from build123d import *

# Parameters (mm, degrees)
PAD001_DEPTH  = 1
PAD_DEPTH     = 5
SKETCH002_R   = 4.25
SKETCH002_R_2 = 3
SKETCH002_W   = 3
SKETCH002_H   = 16
POCKET_DEPTH  = 5


with BuildPart() as part:
    # Sketch → Pad001 (new body)
    with BuildSketch(Plane.XY):
        with BuildLine():
            Line((0, 67), (0, 0))
            Line((0, 0), (55.315734, 3.5))
            ThreePointArc((55.315734, 3.5), (58.645454, 5.067936), (60, 8.490021))
            Line((60, 8.490021), (60, 58.509979))
            ThreePointArc((60, 58.509979), (58.645454, 61.932064), (55.315734, 63.5))
            Line((55.315734, 63.5), (0, 67))
        make_face()
    extrude(amount=PAD001_DEPTH)

    # Sketch001 → Pad (join)
    with BuildSketch(Plane.XY):
        Polygon((1.5, 65.5), (4.5, 65.5), (56, 58.5), (56, 8.5), (3.5, 1.5), (1.5, 1.5), align=None)
        Polygon((3.5, 63.5), (3.5, 3.5), (54, 10.5), (54, 56.5), align=None, mode=Mode.SUBTRACT)
    extrude(amount=PAD_DEPTH)

    # Sketch002 → Pocket (cut, symmetric)
    with BuildSketch(Plane.XY):
        with Locations((40, 33)):
            Circle(SKETCH002_R)
        with Locations((16.5, 20)):
            Circle(SKETCH002_R_2)
        with Locations((16.5, 48)):
            Rectangle(SKETCH002_W, SKETCH002_H)
    extrude(amount=POCKET_DEPTH, both=True, mode=Mode.SUBTRACT)


solid = part.part
The listing builds one solid part. Answer for the finished solid, in the listing's coordinates (mm). A direction names the side the tool comes from. Round coordinates to 2 decimals unless told otherwise and drop trailing zeros. Order: outer loops, then holes, each group sorted by start corner. A loop starts at its lowest first (then second) coordinate and runs counter-clockwise, first axis right, second up. Notation, with made-up numbers: M 50.5,75.25 L 89.5,75.25 A13 cw 89.5,83.25 Z; hole C 47.25,86.25 d2. An arc over 180 degrees is marked long. Answer in a Markdown table with one row per item. Add a question column.
1) The part is cut by section B-B on z = 3.2. Determine the outline of the cut face in (x, y).
2) The part is cut by section D-D on y = 25. Determine the outline of the cut face in (x, z).
3) Determine the mould class of faces 6 (the face through (3.5, 34, 3)), 7 (the face through (3, 34, 5)), 8 (the face through (29.89, 62.05, 2.97)), 9 (the face through (14.1, 18.2, 0.5)) for opening direction X: pulls with the +X half, pulls with the -X half, needs draft (parallel to the pull), parting line crosses it, or undercut.
4) The part is cut by section C-C on x = 40. Determine the outline of the cut face in (y, z), plus the area to 3 significant figures.
5) Consider line 1 along X through (y, z) = (33, 0.8); line 2 along X through (y, z) = (20, 0.55); line 3 along Y through (x, z) = (16.5, 0.55). Determine where each line is inside the solid, lowest interval first. Write a range as from..to.
6) Flat-ended cylindrical pins translate along their axes: pin 1 Ø0.8 at (x, z) = (16.5, 0.5) entering from -Y; pin 2 Ø7 at (x, y) = (16.5, 20) entering from +Z; pin 3 Ø2 at (y, z) = (42, 3.5) entering from +X. Find the tip coordinate at first contact, or state that the pin passes through.
7) The part is cut by section A-A on y = 33. Determine the outline of the cut face in (x, z).
8) Which of the six approach directions +Z, -Z, +X, -X, +Y, -Y give full straight-line access (tool end or side, diameter ignored) to faces 1 (the face through (3, 65.5, 3)), 2 (the face through (56, 34, 3)), 3 (the face through (3, 1.5, 3)), 4 (the face through (1.5, 33, 3)), 5 (the face through (28, 34, 1))?
Findings below:
| question | item | result |
|---|---|---|
| 1 | outline | M 1.5,1.5 L 3.5,1.5 L 56,8.5 L 56,58.5 L 4.5,65.5 L 1.5,65.5 Z; hole M 3.5,3.5 L 54,10.5 L 54,56.5 L 3.5,63.5 Z |
| 2 | outline | M 0,0 L 60,0 L 60,1 L 56,1 L 56,5 L 54,5 L 54,1 L 3.5,1 L 3.5,5 L 1.5,5 L 1.5,1 L 0,1 Z |
| 3 | face 6 | undercut |
| 3 | face 7 | needs draft |
| 3 | face 8 | pulls with the +X half |
| 3 | face 9 | undercut |
| 4 | outline | M 2.53,0 L 28.75,0 L 28.75,1 L 8.56,1 L 8.56,5 L 6.37,5 L 6.37,1 L 2.53,1 Z; M 37.25,0 L 64.47,0 L 64.47,1 L 60.67,1 L 60.67,5 L 58.44,5 L 58.44,1 L 37.25,1 Z |
| 4 | area | 71.1 mm² |
| 5 | line 1 | x = 0..35.75, 44.25..60 |
| 5 | line 2 | x = 0..13.5, 19.5..60 |
| 5 | line 3 | y = 1.04..17, 23..40, 56..65.96 |
| 6 | pin 1 | stops at y = 1.02 |
| 6 | pin 2 | stops at z = 1 |
| 6 | pin 3 | stops at x = 56 |
| 7 | outline | M 0,0 L 35.75,0 L 35.75,1 L 3.5,1 L 3.5,5 L 1.5,5 L 1.5,1 L 0,1 Z; M 44.25,0 L 60,0 L 60,1 L 56,1 L 56,5 L 54,5 L 54,1 L 44.25,1 Z |
| 8 | face 1 | +Z, +X, -X, +Y |
| 8 | face 2 | +Z, +X, +Y, -Y |
| 8 | face 3 | +Z, +X, -X, -Y |
| 8 | face 4 | +Z, -X, +Y, -Y |
| 8 | face 5 | +Z |
